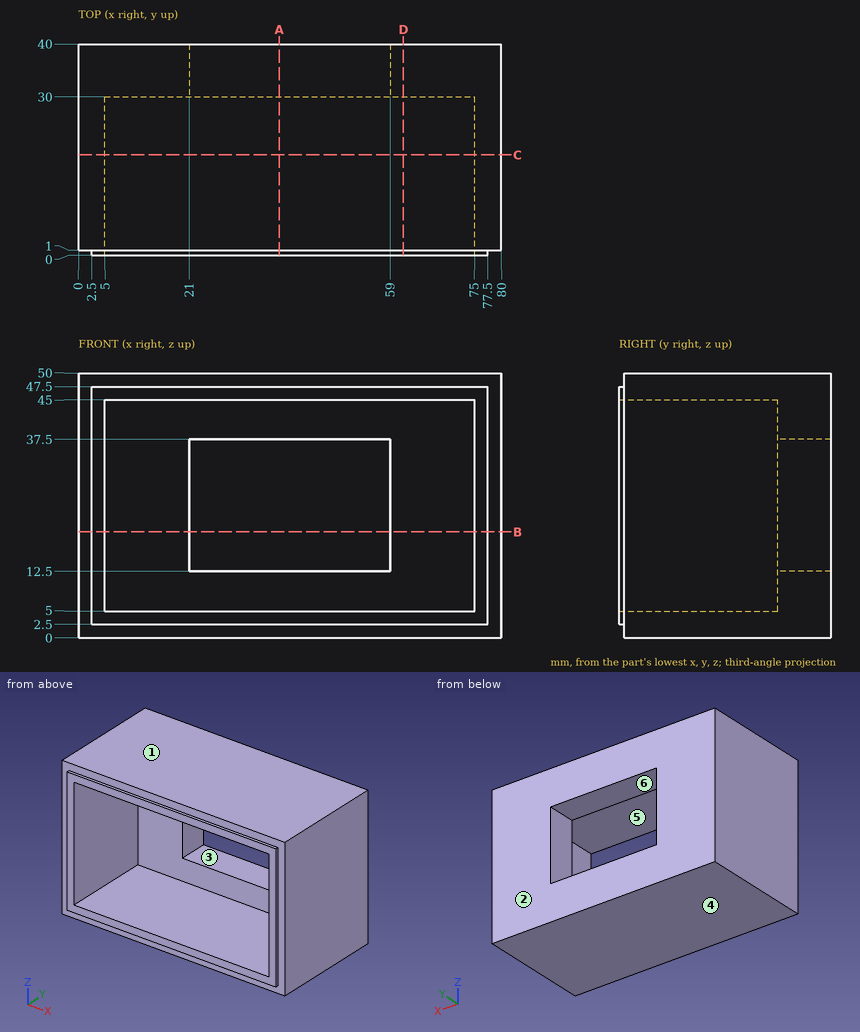
Verification items for this drawing (mm, ordinates from the low corner). A direction names the side the tool comes from. Give positions to 0.01 mm unless a question says otherwise; leave off trailing zeros. Write each loop counter-clockwise with the first axis right and the second up, starting at its lowest first coordinate (ties: lowest second). Pieces come first, ordered by that corner, then holes.
1) Cross-section at A-A (x = 38). Record the boundary of the cut face in (y, z), plus the area to 3 significant figures.
Values follow:
outline: (0, 2.5) - (1, 2.5) - (1, 0) - (40, 0) - (40, 12.5) - (30, 12.5) - (30, 5) - (0, 5) - close; (0, 45) - (30, 45) - (30, 37.5) - (40, 37.5) - (40, 50) - (1, 50) - (1, 47.5) - (0, 47.5) - close
area: 545 mm2
2) Cross-section at C-C (y = 19). Record the boundary of the cut face in (x, z), plus the area to 3 significant figures.
Values follow:
outline: (0, 0) - (80, 0) - (80, 50) - (0, 50) - close; hole (5, 5) - (75, 5) - (75, 45) - (5, 45) - close
area: 1,200 mm2
3) Go/stop test with flat-tipped pins: pin 1 Ø0.8 at (x, y) = (25, 0.5) entering from +Z; pin 2 Ø12 at (x, z) = (15.5, 17.5) entering from -Y; pin 3 Ø0.5 at (y, z) = (0.5, 29) entering from +X. Record where each tip stops, or that it passes through.
Values follow:
pin 1: stops at z = 47.5
pin 2: stops at y = 30
pin 3: stops at x = 77.5
4) Thickness scan on line 1 (Z direction, x = 45, y = 31); line 2 (X direction, y = 26, z = 6.5); line 3 (X direction, y = 33.5, z = 16.5). Record the ranges inside material, lowest first.
Values follow:
line 1: z = 0 to 12.5, 37.5 to 50
line 2: x = 0 to 5, 75 to 80
line 3: x = 0 to 21, 59 to 80
5) Cross-section at B-B (z = 20). Record the boundary of the cut face in (x, y), plus the area to 3 significant figures.
Values follow:
outline: (0, 1) - (2.5, 1) - (2.5, 0) - (5, 0) - (5, 30) - (21, 30) - (21, 40) - (0, 40) - close; (59, 30) - (75, 30) - (75, 0) - (77.5, 0) - (77.5, 1) - (80, 1) - (80, 40) - (59, 40) - close
area: 715 mm2
6) Release check for a two-part mould opening along Z. For the marked faces 1, 2 and 3 record: released by +Z, released by -Z, zero draft, split by the parting line, or undercut.
Values follow:
face 1: released by +Z
face 2: zero draft
face 3: undercut
7) Set-up check for the marked faces 4, 5 and 6: record each of +Z, -Z, +X, -X, +Y, -Y from which the full face is reachable in a straight line by a thin tool's end or side.
Values follow:
face 4: -Z, +X, -X, +Y, -Y
face 5: -Y
face 6: +Y, -Y
8) Cross-section at D-D (x = 61.5). Record the boundary of the cut face in (y, z), plus the area to 3 significant figures.
Values follow:
outline: (0, 2.5) - (1, 2.5) - (1, 0) - (40, 0) - (40, 50) - (1, 50) - (1, 47.5) - (0, 47.5) - (0, 45) - (30, 45) - (30, 5) - (0, 5) - close
area: 795 mm2
